For this review, take the finished solid that the model builds, in its own axes (mm). Face numbers are marked on the shaded views. A direction names the side the tool comes from. Round coordinates to 2 decimals unless told otherwise and drop trailing zeros. Order: outer loops, then holes, each group sorted by start corner. A loop starts at its lowest first (then second) coordinate and runs counter-clockwise, first axis right, second up. Notation, with made-up numbers: M 34.25,-6.5 L 75.25,-6.5 A10 cw 75.25,8.5 Z; hole C -24,44.5 d7. An arc over 180 degrees is marked long. Answer as a JSON object with one key per item and string values.
from build123d import *

# Parameters (mm, degrees)
F0_R      = 8.125
F1_DEPTH  = 18
F2_SIZE   = 1
F3_R      = 10
F4_DEPTH  = 34.3
F5_R      = 7.95
F6_DEPTH  = 3.4
F8_R      = 10
F9_DEPTH  = 14.3
F10_R     = 8.125
F11_DEPTH = 8
F12_SIZE  = 1
F13_SIZE  = 0.5
F14_R     = 0.3


with BuildPart() as f1:
    # F0 (on Top) → F1 (new body)
    with BuildSketch(Plane.XY):
        Circle(F0_R)
    extrude(amount=F1_DEPTH)

    # F2
    f2_edges = [f1.edges().sort_by_distance(p)[0] for p in [
        (-8.125, 0, 0),
    ]]
    chamfer(f2_edges, length=F2_SIZE)

    # F3 (on face) → F4 (join)
    with BuildSketch(Plane.XY.offset(18)):
        Circle(F3_R)
    extrude(amount=F4_DEPTH)

    # F5 (on face) → F6 (join)
    with BuildSketch(Plane.XY.offset(52.3)):
        Circle(F5_R)
    extrude(amount=F6_DEPTH)

    # F8 (on face) → F9 (join)
    with BuildSketch(Plane.XY.offset(55.7)):
        Circle(F8_R)
    extrude(amount=F9_DEPTH)

    # F10 (on face) → F11 (join)
    with BuildSketch(Plane.XY.offset(70)):
        Circle(F10_R)
    extrude(amount=F11_DEPTH)

    # F12
    f12_edges = [f1.edges().sort_by_distance(p)[0] for p in [
        (-8.125, 0, 78),
    ]]
    chamfer(f12_edges, length=F12_SIZE)

    # F13
    f13_edges = [f1.edges().sort_by_distance(p)[0] for p in [
        (-10, 0, 70),
    ]]
    chamfer(f13_edges, length=F13_SIZE)

    # F14
    f14_edges = [f1.edges().sort_by_distance(p)[0] for p in [
        (-10, 0, 55.7),
        (-10, 0, 52.3),
    ]]
    fillet(f14_edges, radius=F14_R)


solid = f1.part
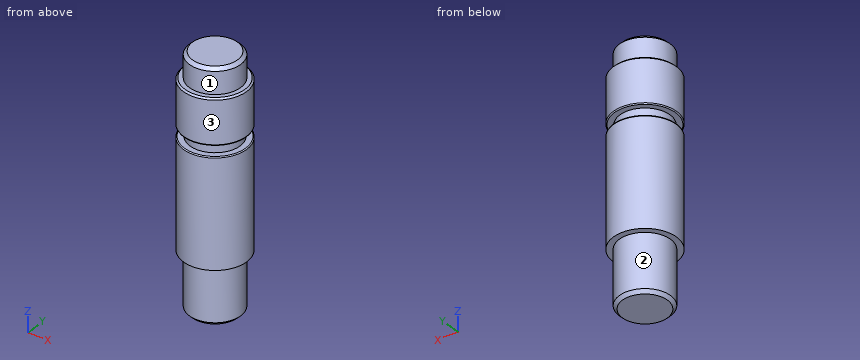
1) Machinability: for the marked faces 1, 2 and 3, which of the approach directions +Z, -Z, +X, -X, +Y, -Y give a long, thin tool a straight path to every point of the face, cutting with its end or side? Answer none if there is none.
Geometry check:
{"face 1": "+Z", "face 2": "-Z", "face 3": "+Z, -Z"}
2) Add section D-D on z = 43. State the section outline as (x, y) points.
Geometry check:
{"outline": "C 0,0 d20"}
3) Insertion check: P1, Ø5, axis at x = -2.5, z = 13.5, coming from the -Y side (3 decimals); P2, Ø6, axis at y = -7.5, z = 17, coming from the +X side; P3, Ø1, axis at x = -1.5, z = 32, coming from the +Y side. Each pin has a flat end and moves straight along its axis. Give the tip position at first contact, or say it passes through.
Geometry check:
{"P1": "stops at y = -8.125", "P2": "stops at x = 8.84", "P3": "stops at y = 9.95"}
4) For L1, parallel to Z at x = -3.25, y = 8.5; L2, parallel to X at y = 0.5, z = 18.5; L3, parallel to X at y = 0.25, z = 16, list the stretches that pass through material, from the lowest coordinate up.
Geometry check:
{"L1": "z = 18 to 52.3, 55.7 to 70", "L2": "x = -9.99 to 9.99", "L3": "x = -8.12 to 8.12"}
5) Add section C-C on z = 71. State the section outline as (x, y) points (3 decimals), and give its area (3 significant figures).
Geometry check:
{"outline": "C 0,0 d16.25", "area": "207 mm²"}
